Autodesk Inventor part; units mm, degrees
ref_plane "YZ Plane" through (0, 0, 0) normal (1, 0, 0) x (0, 1, 0)
ref_plane "XZ Plane" through (0, 0, 0) normal (0, 1, 0) x (-1, 0, 0)
ref_plane "XY Plane" through (0, 0, 0) normal (0, 0, 1) x (1, 0, 0)
sketch "草圖1" plane through (0, 0, 0) normal (0, 1, 0) x (-1, 0, 0)
  line L0 (71.0233, 6.25) -> (1.0233, 6.25)
  line L1 (1.0233, 6.25) -> (1.0233, -6.25)
  line L2 (1.0233, -6.25) -> (71.0233, -6.25)
  line L3 (71.0233, -6.25) -> (71.0233, 6.25)
  line L4 (1.0233, 5) -> (-4.9767, 5)
  line L5 (-4.9767, 5) -> (-4.9767, 7.5)
  line L6 (-4.9767, 7.5) -> (1.0233, 7.5)
  line L7 (1.0233, 7.5) -> (1.0233, 5)
  line L8 (1.0233, -5) -> (-4.9767, -5)
  line L9 (-4.9767, -5) -> (-4.9767, -7.5)
  line L10 (-4.9767, -7.5) -> (1.0233, -7.5)
  line L11 (1.0233, -7.5) -> (1.0233, -5)
  point P0 (0, 0)
  point P1 (1.0233, 6.25)
  dimension "d0" = 6
  dimension "d2" = 5
  dimension "d3" = 10
  dimension "d4" = 2.5
  dimension "d5" = 12.5
  dimension "d6" = 6.25
  dimension "d7" = 70
extrude "擠出1" add sketch "草圖1" along normal mid plane 10
sketch "草圖2" plane through (-1.0233, 5, 7.5) normal (0, 0, 1) x (1, 0, 0)
  line L0 (6, -10) -> (6, 0)
  circle A0 centre (6, -5) radius 1.5
  point P0 (1.0233, -5)
  dimension "d10" = 3
extrude "擠出2" add sketch "草圖2" against normal up to surface (15 mm away)
sketch "草圖3" plane through (4.9767, 5, 7.5) normal (1, 0, 0) x (0, 0, -1)
  line L0 (15, -10) -> (12.5, -10)
  circle A0 centre (7.5, -5) radius 9.0139
  circle A1 centre (7.5, -5) radius 10.7008
  line L1 (15, -3.5) -> (15, 0)
  line L2 (15, -10) -> (15, 0)
  line L3 (2.5, -10) -> (0, -10)
  line L4 (0, -3.5) -> (0, 0)
  line L5 (0, -10) -> (0, 0)
extrude "擠出3" add sketch "草圖3" against normal up to surface (6 mm away) contours A0 L2 L1 | L4 L5 A0 | A1
properties part number "axis_rf"
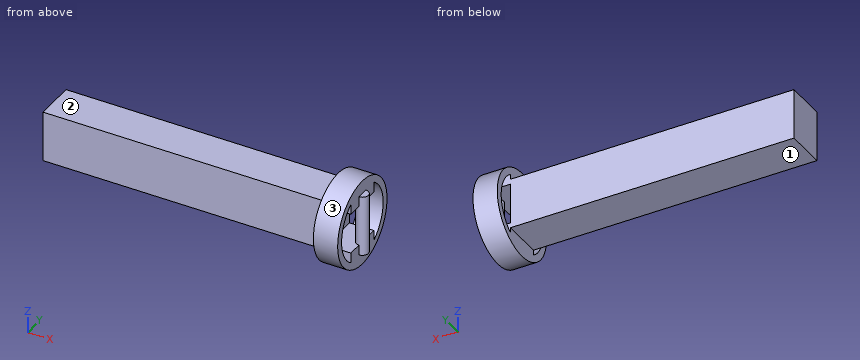
CAD build for the part. Positions are in the model's coordinates, mm. Face numbers are marked on the shaded views. A direction names the side the tool comes from. Round coordinates to 2 decimals unless told otherwise and drop trailing zeros. Write each loop counter-clockwise with the first axis right and the second up, starting at its lowest first coordinate (ties: lowest second). Pieces come first, ordered by that corner, then holes. Notation, with made-up numbers: (16, 44) -> (47, 44) arc R11 ccw to (47, 52) -> close; hole circle Ø8 at (-33.75, -13). An arc over 180 degrees is marked (long way). Answer in a Markdown table with one row per item. Add a question column.
Item 1: Saw through at C-C, the plane x = 0.5. Write the cut outline in (y, z), then the cut area to 3 significant figures.
Item 2: Saw through at B-B, the plane y = 0. Write the cut outline in (x, z), then the cut area to 3 significant figures.
Item 3: Drop flat-ended pins along their axis: pin 1 Ø12 at (x, z) = (-19.5, 1.5) entering from +Y; pin 2 Ø12 at (x, z) = (-41, 2.5) entering from -Y; pin 3 Ø2 at (y, z) = (6.5, 1.5) entering from +X; pin 4 Ø3 at (x, y) = (-51.5, 0) entering from +Z. Give the stop position or say it passes through.
Item 4: Drill centre lines: line 1 (X direction, y = 4.25, z = 9.25); line 2 (Y direction, x = -34, z = 5.5); line 3 (Z direction, x = -34.5, y = -4.5). Where is each one in solid material? Low to high. Write a range as from..to.
Item 5: Which spindle directions (+Z, -Z, +X, -X, +Y, -Y) get a long thin tool onto all of the face, cutting with end or side? Do the marked faces 1, 2 and 3. Say none if no direction does.
Item 6: Saw through at A-A, the plane z = 0. Write the cut outline in (x, y), then the cut area to 3 significant figures.
Item 7: Saw through at D-D, the plane y = -8.25. Write the cut outline in (x, z).
Findings below:
| question | item | result |
|---|---|---|
| 1 | outline | circle Ø21.4 at (0, 0); hole (-5, -7.5) -> (-5, -5) -> (5, -5) -> (5, -7.5) arc R9.01 ccw to (5, 7.5) -> (5, 5) -> (-5, 5) -> (-5, 7.5) arc R9.01 ccw to start |
| 1 | area | 175 mm^2 |
| 2 | outline | (-71.02, -6.25) -> (-1.02, -6.25) -> (-1.02, -10.7) -> (4.98, -10.7) -> (4.98, -7.5) -> (6.48, -7.5) -> (6.48, 7.5) -> (4.98, 7.5) -> (4.98, 10.7) -> (-1.02, 10.7) -> (-1.02, 6.25) -> (-71.02, 6.25) -> close; hole (-1.02, -5) -> (3.48, -5) -> (3.48, 5) -> (-1.02, 5) -> close |
| 2 | area | 981 mm^2 |
| 3 | pin 1 | stops at y = 5 |
| 3 | pin 2 | stops at y = -5 |
| 3 | pin 3 | passes through |
| 3 | pin 4 | stops at z = 6.25 |
| 4 | line 1 | x = -1.02..4.98 |
| 4 | line 2 | y = -5..5 |
| 4 | line 3 | z = -6.25..6.25 |
| 5 | face 1 | -Z, -X, +Y, -Y |
| 5 | face 2 | +Z, -X, +Y, -Y |
| 5 | face 3 | +X, -X |
| 6 | outline | (-71.02, -5) -> (-1.02, -5) -> (-1.02, 5) -> (-71.02, 5) -> close; (-1.02, -10.7) -> (4.98, -10.7) -> (4.98, -9.01) -> (-1.02, -9.01) -> close; (-1.02, 9.01) -> (4.98, 9.01) -> (4.98, 10.7) -> (-1.02, 10.7) -> close; circle Ø3 at (4.98, 0) |
| 6 | area | 727 mm^2 |
| 7 | outline | (-1.02, -6.82) -> (4.98, -6.82) -> (4.98, -3.63) -> (-1.02, -3.63) -> close; (-1.02, 3.63) -> (4.98, 3.63) -> (4.98, 6.82) -> (-1.02, 6.82) -> close |
